from build123d import *

# Parameters (mm, degrees)
SKETCH_1_R      = 3
EXTRUDE_1_DEPTH = 2.5
FILLET_1_R      = 0.05
FILLET_2_R      = 0.05


with BuildPart() as part:
    # Эскиз1 → Бобышка-Вытянуть1 (new body)
    with BuildSketch(Plane(origin=(0, 0, 0), x_dir=(1, 0, 0), z_dir=(0, 1, 0))):
        with Locations(Location((0, 0, 0), (0, 0, 270))):
            Circle(SKETCH_1_R)
    extrude(amount=EXTRUDE_1_DEPTH)

    # Скругление1
    fillet_1_edges = [part.edges().sort_by_distance(p)[0] for p in [
        (0, 2.5, -3),
    ]]
    fillet(fillet_1_edges, radius=FILLET_1_R)

    # Скругление2
    fillet_2_edges = [part.edges().sort_by_distance(p)[0] for p in [
        (0, 0, -3),
    ]]
    fillet(fillet_2_edges, radius=FILLET_2_R)


solid = part.part
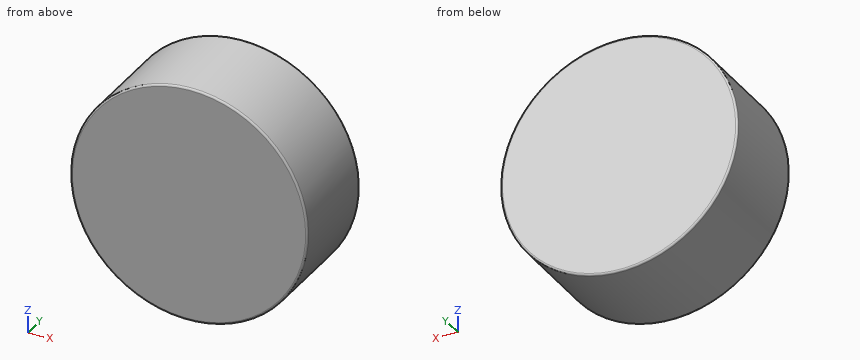
Source: CAD feature listing. Evaluate the final solid. Frame: model axes, mm. Round coordinates to 2 decimals unless told otherwise and drop trailing zeros. Loops run counter-clockwise (first coordinate to the right, second up) from the corner with the lowest first, then second, coordinate; pieces in that order, holes last. Notation, with made-up numbers: (15, -11) -> (55, -11) arc R4 ccw to (55, -6) -> close; hole circle Ø7 at (14, 7.25). An arc over 180 degrees is marked (long way). Answer as a JSON object with one key per item and string values. Group by question number.
Q1. Contact query for flat-ended pins moving along their axis: P1, Ø1, axis at x = -1.5, y = 1, coming from the +Z side; P2, Ø1.5, axis at x = 1.5, y = 0.5, coming from the -Z side; P3, Ø1, axis at y = 2, z = -1.5, coming from the -X side. Output: stop coordinate, or through.
Q2. Ray query, line 1 (Z direction, x = -1.25, y = 1.75); line 2 (X direction, y = 1.5, z = -0.25); line 3 (Z direction, x = 1.5, y = 1.5). Return the intervals inside material, ascending. Write a range as from..to.
Q3. Section query A-A (y = 1.85). Output: boundary loops of the cut face in (x, z).
Completed:
{
 "1": {"P1": "z = 2.83", "P2": "z = -2.9", "P3": "x = -2.83"},
 "2": {"line 1": "-2.73..2.73", "line 2": "-2.99..2.99", "line 3": "-2.6..2.6"},
 "3": {"outline": "circle Ø6 at (0, 0)"}
}
